Check sheet for the modelled part. Datum: model origin and axes. Units: mm. Face numbers are marked on the shaded views. A direction names the side the tool comes from. Round coordinates to 2 decimals unless told otherwise and drop trailing zeros. Order: outer loops, then holes, each group sorted by start corner. A loop starts at its lowest first (then second) coordinate and runs counter-clockwise, first axis right, second up. Notation, with made-up numbers: (54, 77.5) -> (94, 77.5) arc R24 cw to (94, 112.5) -> close; hole circle Ø10 at (33.5, -34). An arc over 180 degrees is marked (long way). Use CSV: the item, a comma, the result in double quotes.
Autodesk Fusion 360 part; units mm, degrees
sketch "Sketch1" plane through (0, 0, 0) normal (0, 0, 1) x (1, 0, 0)
  line L0 (0, 0) -> (30, 0)
  line L1 (30, 0) -> (30, 15)
  line L2 (30, 15) -> (0, 15)
  line L3 (0, 15) -> (0, 0)
  circle A0 centre (15, 7.5) radius 1
  line L4 (0, 0) -> (30, 0)
  line L5 (30, 0) -> (30, -5)
  line L6 (30, -5) -> (0, -5)
  line L7 (0, -5) -> (0, 0)
  dimension "d1" = 30
  dimension "d2" = 15
  dimension "d3" = 2
  dimension "d4" = 7.5
  dimension "d5" = 15
  dimension "d6" = 5
extrude "Extrude1" add sketch "Sketch1" along normal blind 10
extrude "Extrude2" add sketch "Sketch1" against normal blind 15 contours L0 L4 L5 L6 L7
fillet "Fillet1" radius 3.5 2 edges at (15, 15, 10) (15, 15, 0)
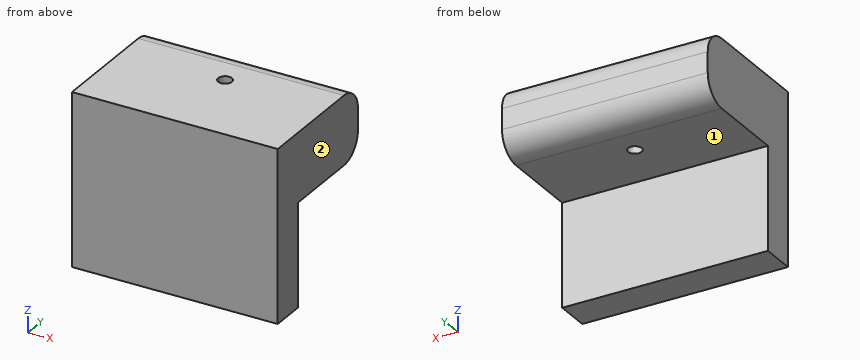
Q1. Sectioned sample at A-A, the plane y = 7.5. Enter the section's corners in (x, z).
Result sheet:
outline,"(0, 0) -> (14, 0) -> (14, 10) -> (0, 10) -> close; (16, 0) -> (30, 0) -> (30, 10) -> (16, 10) -> close"
Q2. Sectioned sample at D-D, the plane z = -0.5. Enter the section's corners in (x, y), then the cut area to 3 significant figures.
Result sheet:
outline,"(0, -5) -> (30, -5) -> (30, 0) -> (0, 0) -> close"
area,"150 mm^2"
Q3. Go/stop test with flat-tipped pins: pin 1 (10 mm diameter, centred on x = 22, y = 5.5, fed in from -Z); pin 2 (2 mm diameter, centred on x = 18, z = -9, fed in from +Y); pin 3 (1.8 mm diameter, centred on x = 15, y = 7.5, fed in from +Z). Record where each tip stops, or that it passes through.
Result sheet:
pin 1,"stops at z = 0"
pin 2,"stops at y = 0"
pin 3,"passes through"
Q4. Scan lines: L1, parallel to Y at x = 15, z = 5.5; L2, parallel to Z at x = 12.5, y = 3; L3, parallel to Y at x = 12.5, z = -6. Record each from-to range of solid material in increasing order.
Result sheet:
L1,"y = -5 to 6.5, 8.5 to 15"
L2,"z = 0 to 10"
L3,"y = -5 to 0"
Q5. Access from +Z, -Z, +X, -X, +Y, -Y to the whole of each face (thin tool, end or side, straight path). Record for the marked faces 1 and 2.
Result sheet:
face 1,"-Z, +X, -X, +Y"
face 2,"+Z, -Z, +X, +Y, -Y"
Q6. Sectioned sample at C-C, the plane x = 24. Enter the section's corners in (y, z).
Result sheet:
outline,"(-5, -15) -> (0, -15) -> (0, 0) -> (11.5, 0) arc R3.5 ccw to (15, 3.5) -> (15, 6.5) arc R3.5 ccw to (11.5, 10) -> (-5, 10) -> close"
Q7. Sectioned sample at B-B, the plane x = 15. Enter the section's corners in (y, z), then the cut area to 3 significant figures.
Result sheet:
outline,"(-5, -15) -> (0, -15) -> (0, 0) -> (6.5, 0) -> (6.5, 10) -> (-5, 10) -> close; (8.5, 0) -> (11.5, 0) arc R3.5 ccw to (15, 3.5) -> (15, 6.5) arc R3.5 ccw to (11.5, 10) -> (8.5, 10) -> close"
area,"250 mm^2"
